```python
from build123d import *

# Parameters (mm, degrees)
BOSS_EXTRUDE1_DEPTH = 18.161
CUT_EXTRUDE1_DEPTH  = 24.638
CUT_EXTRUDE2_DEPTH  = 19.05
CRVPATTERN1_START   = -0.889
CRVPATTERN1_DEPTH   = 19.05


# Read off the part's stored shape, not the designer's step: CrvPattern1
with BuildPart() as part:
    # Sketch1 → Boss-Extrude1 (new, symmetric)
    with BuildSketch(Plane(origin=(0, 0, 0), x_dir=(1, 0, 0), z_dir=(0, 1, 0))):
        with BuildLine():
            Line((0, 66.607667907), (0, -265.604400607))
            ThreePointArc((0, -265.604400607), (-78.340784416, -202.581490406), (-45.87811803, -107.421934899))
            ThreePointArc((-45.87811803, -107.421934899), (-40.160322886, -75.527015006), (-51.603877928, -45.211604003))
            ThreePointArc((-51.603877928, -45.211604003), (-60.864208699, 26.879044906), (0, 66.607667907))
        make_face()
    boss_extrude1 = extrude(amount=BOSS_EXTRUDE1_DEPTH, both=True)

    # Mirror1: Boss-Extrude1 across plane
    add(boss_extrude1.mirror(Plane(origin=(0, 0, 0), x_dir=(0, 0, 1), z_dir=(1, 0, 0))))

    # Sketch2 → Cut-Extrude1 (cut)
    with BuildSketch(Plane(origin=(0, 18.161, 0), x_dir=(1, 0, 0), z_dir=(0, 1, 0))):
        with BuildLine():
            ThreePointArc((0, 41.200992494), (-38.018423714, 15.7584639), (-31.604351091, -29.535933937))
            ThreePointArc((-31.604351091, -29.535933937), (-14.627606963, -76.491037862), (-26.48852554, -124.99165885))
            ThreePointArc((-26.48852554, -124.99165885), (-54.824707805, -192.124773269), (0, -240.125249216))
            ThreePointArc((0, -240.125249216), (54.824707805, -192.124773269), (26.48852554, -124.99165885))
            ThreePointArc((26.48852554, -124.99165885), (14.627606963, -76.491037862), (31.604351091, -29.535933937))
            ThreePointArc((31.604351091, -29.535933937), (38.018423714, 15.7584639), (0, 41.200992494))
        make_face()
    extrude(amount=-CUT_EXTRUDE1_DEPTH, mode=Mode.SUBTRACT)

    # Sketch3 → Cut-Extrude2 (cut)
    with BuildSketch(Plane(origin=(0, 18.161, 0), x_dir=(1, 0, 0), z_dir=(0, 1, 0))):
        Polygon((10.046315092, 53.239317383), (5.023157546, 61.939681467), (-5.023157546, 61.939681467), (-10.046315092, 53.239317383), (-5.023157546, 44.538953299), (5.023157546, 44.538953299), align=None)
    extrude(amount=-CUT_EXTRUDE2_DEPTH, mode=Mode.SUBTRACT)

    # CrvPattern1 outline → CrvPattern1 (cut)
    with BuildSketch(Plane(origin=(0, 0, 0), x_dir=(1, 0, 0), z_dir=(0, 1, 0)).offset(CRVPATTERN1_START)):
        Polygon((37.533514674, -27.403244166), (31.332053305, -35.307061206), (35.076228964, -44.629592813), (45.021865992, -46.048307379), (51.223327362, -38.144490339), (47.479151703, -28.821958732), align=None)
        Polygon((44.628135866, 5.689936437), (45.431707419, -4.32418957), (54.505980714, -8.635339196), (62.776682456, -2.932362814), (61.973110904, 7.081763193), (52.898837609, 11.392912818), align=None)
        Polygon((27.396514919, 34.820049581), (34.77897318, 28.006257908), (44.371118995, 30.992758468), (46.580806549, 40.7930507), (39.198348288, 47.606842373), (29.606202473, 44.620341813), align=None)
    extrude(amount=CRVPATTERN1_DEPTH, mode=Mode.SUBTRACT)


solid = part.part
```
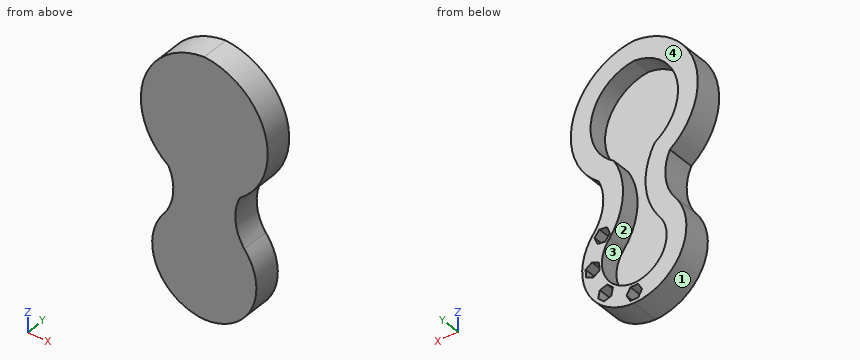
For this review, take the finished solid that the model builds, in its own axes (mm). Face numbers are marked on the shaded views. A direction names the side the tool comes from. Coordinates: 2 decimals unless noted, no trailing zeros. Loops run counter-clockwise (first coordinate to the right, second up) from the corner with the lowest first, then second, coordinate; pieces in that order, holes last. Notation, with made-up numbers: (-4.5, 65.25) - (46.5, 65.25) arc R24 cw to (46.5, 98.25) - close; hole circle Ø9 at (-9, 6). An arc over 180 degrees is marked (long way). Use one line per item in the form item = value. Start each with the question number.
1) Draft analysis for pull direction Z (two halves, no side actions). For the marked faces 3 and 4, state which applies: released by +Z, released by -Z, zero draft, split by the parting line, or undercut.
2) Take a section at A-A (z = 20). State the section outline as (x, y) points, plus the area to 3 significant figures.
3) To check wall thickness, follow probe 1 along Z at (x, y) = (25, -5); probe 2 along Z at (x, y) = (38.5, 1); probe 3 along X at (y, z) = (10, 42.5). State the ranges of each line that lie inside material, in increasing order. Write a range as from..to.
4) For pin 1 (10 mm diameter, centred on y = 6, z = -11.5, fed in from +X); pin 2 (5 mm diameter, centred on x = 56.5, y = 13, fed in from -Z); pin 3 (1.5 mm diameter, centred on x = -10.5, y = 7.5, fed in from -Z), all flat-tipped, find the tip position at first contact; note any pin that passes through.
5) Take a section at B-B (y = 9). State how many separate pieces and enclosed holes the cut face has, plus the area to 3 significant figures.
6) Take a section at C-C (z = 97.5). State the section outline as (x, y) points.
7) For the marked faces 1 and 2, list the 3-axis set-ups (+Z, -Z, +X, -X, +Y, -Y) from which the entire face can be reached by the end or side of a thin tool; tool diameter is ignored.
From the geometry:
q1.face_3 = undercut
q1.face_4 = zero draft
q2.outline = (-64.69, -18.16) - (64.69, -18.16) - (64.69, 18.16) - (37.71, 18.16) - (37.71, -6.48) - (-37.71, -6.48) - (-37.71, 18.16) - (-64.69, 18.16) - close
q2.area = 2,840 mm2
q3.probe_1 = -61.38..-32.28, 39.86..122.37, 232.23..260.2
q3.probe_2 = -53.89..-47.39, -29.16..-14.64, 18.2..27.54, 45.12..134.49, 221.85..253.77
q3.probe_3 = -53.72..-23.62, 23.62..34.22, 47.81..53.72
q4.pin_1 = 66.66
q4.pin_2 = -38.55
q4.pin_3 = -65.73
q5.separate_pieces = 1
q5.enclosed_holes = 5
q5.area = 18,900 mm2
q6.outline = (-42.15, -18.16) - (42.15, -18.16) - (42.15, 18.16) - (16.07, 18.16) - (16.07, -6.48) - (-16.07, -6.48) - (-16.07, 18.16) - (-42.15, 18.16) - close
q7.face_1 = -X, +Y, -Y
q7.face_2 = +Y
